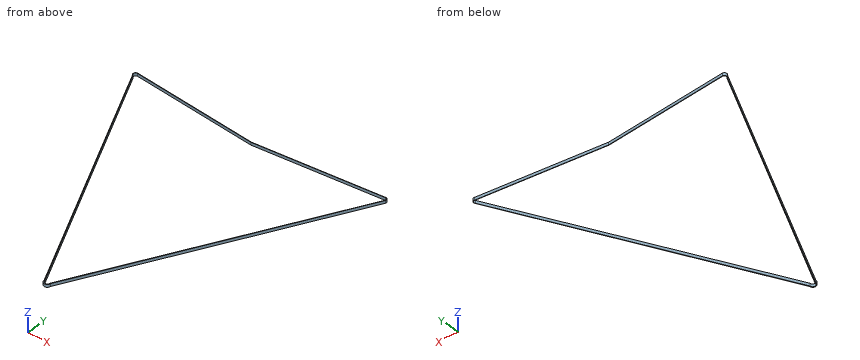
Autodesk Inventor part; units mm, degrees
ref_plane "YZ Plane" through (0, 0, 0) normal (1, 0, 0) x (0, 1, 0)
ref_plane "XZ Plane" through (0, 0, 0) normal (0, 1, 0) x (-1, 0, 0)
ref_plane "XY Plane" through (0, 0, 0) normal (0, 0, 1) x (1, 0, 0)
sketch "Sketch1" plane through (0, 0, 0) normal (0, 0, 1) x (1, 0, 0)
  arc A0 (-287.0527, -558.563) -> (-272.0536, -558.5587) centre (-279.5531, -558.6452) ccw
  line L0 (-561.7795, -4.4916) -> (-287.0527, -558.563)
  line L1 (-272.0536, -558.5587) -> (6.4474, -0.1094)
  line L2 (-0.0123, 6.4539) -> (-558.6713, 5.3904)
  arc A1 (-558.6713, 5.3904) -> (-561.7795, -4.4916) centre (-558.6609, -0.0427) ccw
  arc A2 (6.4474, -0.1094) -> (-0.0123, 6.4539) centre (1.1622, 1.1493) ccw
  point P0 (0, 0)
  dimension "d0" = 5.433
extrude "Extrusion1" add sketch "Sketch1" along normal blind 6
sketch "Sketch3" plane through (0, 0, 6) normal (0, 0, 1) x (1, 0, 0)
  line L0 (-561.7795, -4.4916) -> (-287.0527, -558.563)
  arc A0 (-287.0527, -558.563) -> (-272.0536, -558.5587) centre (-279.5531, -558.6452) ccw
  line L1 (-272.0536, -558.5587) -> (6.4474, -0.1094)
  arc A1 (6.4474, -0.1094) -> (-0.0123, 6.4539) centre (1.1622, 1.1493) ccw
  line L2 (-0.0123, 6.4539) -> (-558.6713, 5.3904)
  arc A2 (-558.6713, 5.3904) -> (-561.7795, -4.4916) centre (-558.6609, -0.0427) ccw
  line L3 (-0.0123, 6.4539) -> (-279.291, -20.76)
  line L4 (-0.0123, 6.4539) -> (-558.6713, 5.3904)
  line L5 (-279.291, -20.76) -> (-558.6713, 5.3904)
  line L6 (-558.6713, 5.3904) -> (-279.551, 142.5192)
  line L7 (-279.551, 142.5192) -> (-0.0123, 6.4539)
  point P0 (0, 0)
extrude "Extrusion2" cut sketch "Sketch3" against normal blind 6 contours L6 L7 L2 | L2 L3 L5
sketch "Sketch4" plane through (0, 0, 6) normal (0, 0, 1) x (1, 0, 0)
  point P0 (0, 0)
sketch "Sketch5" plane through (0, 0, 6) normal (0, 0, 1) x (1, 0, 0)
  line L0 (-0.0123, 6.4539) -> (-279.291, -20.76)
  line L1 (-279.291, -20.76) -> (-558.6713, 5.3904)
  arc A0 (-558.6713, 5.3904) -> (-561.7795, -4.4916) centre (-558.6609, -0.0427) ccw
  line L2 (-561.7795, -4.4916) -> (-287.0527, -558.563)
  arc A1 (-287.0527, -558.563) -> (-272.0536, -558.5587) centre (-279.5531, -558.6452) ccw
  line L3 (-272.0536, -558.5587) -> (6.4474, -0.1094)
  arc A2 (6.4474, -0.1094) -> (-0.0123, 6.4539) centre (1.1622, 1.1493) ccw
  arc A3 (-285.3025, -558.563) -> (-273.8037, -558.563) centre (-279.5531, -558.6452) ccw
  arc A4 (5.0344, -1.1313) -> (0.2947, 5.5587) centre (1.1622, 1.1493) ccw
  arc A5 (-558.1379, 4.3653) -> (-560.7286, -3.9705) centre (-558.6609, -0.0427) ccw
  line L4 (-560.7286, -3.9705) -> (-285.3025, -558.563)
  line L5 (-273.8037, -558.563) -> (5.0344, -1.1313)
  line L6 (1.1622, 5.6432) -> (-279.5531, -21.7107)
  line L7 (-279.5531, -21.7107) -> (-558.1379, 4.3653)
  point P0 (0, 0)
  dimension "d5" = 11.5
extrude "Extrusion3" cut sketch "Sketch5" against normal blind 6 contours L4 A5 L7 L6 A4 L5 A3
properties part number "z bELT"
The model under review builds one solid part; all positions refer to its coordinate system, in mm. Coordinates: 2 decimals unless noted, no trailing zeros. Order: outer loops, then holes, each group sorted by start corner. A loop starts at its lowest first (then second) coordinate and runs counter-clockwise, first axis right, second up. Notation, with made-up numbers: M 68.5,-16.5 L 78.5,-16.5 A22 ccw 78.5,-0.5 Z; hole C -31.75,-39 d7. An arc over 180 degrees is marked long. One line per question, with ' | ' between items.
(1) For probe 1 along Y at (x, z) = (-272, 2.6); probe 2 along Y at (x, z) = (-294, 1.75); probe 3 along X at (y, z) = (-82, 4.6), list the stretches that pass through material, from the lowest coordinate up. Write a range as from..to.
Geometry results:
probe 1: y = -558.45..-554.96, -20.97..-20.05 | probe 2: y = -544.55..-541.05, -20.36..-19.38 | probe 3: x = -523.35..-521.98, -35.42..-34.39
(2) Add section C-C, the plane y = -111. Write out the cut boundary in (x, z), then the cut area to 3 significant figures.
Geometry results:
outline: M -508.97,0 L -507.57,0 L -507.57,6 L -508.97,6 Z; M -49.92,0 L -48.85,0 L -48.85,6 L -49.92,6 Z | area: 14.8 mm²
(3) Add section B-B, the plane x = -71.5. Write out the cut boundary in (y, z).
Geometry results:
outline: M -156.41,0 L -154.13,0 L -154.13,6 L -156.41,6 Z; M -1.44,0 L -0.51,0 L -0.51,6 L -1.44,6 Z
(4) Add section A-A, the plane z = 2.1. Write out the cut boundary in (x, y), then the cut area to 3 significant figures.
Geometry results:
outline: M -561.78,-4.49 L -287.05,-558.56 A7.5 ccw long -272.05,-558.56 L 6.45,-0.11 A5.43 ccw -0.01,6.45 L -279.29,-20.76 L -558.67,5.39 A5.43 ccw Z; hole M -560.73,-3.97 L -285.3,-558.56 A5.75 ccw long -273.8,-558.56 L 5.03,-1.13 A4.49 ccw 1.16,5.64 L -279.55,-21.71 L -558.14,4.37 A4.44 ccw Z | area: 2,180 mm²
(5) Insertion check: pin 1 (1.5 mm diameter, centred on y = -447.5, z = 4.5, fed in from -X); pin 2 (1 mm diameter, centred on x = -200.5, z = 4.5, fed in from -Y); pin 3 (3 mm diameter, centred on y = -75.5, z = 1.5, fed in from -X). Each pin has a flat end and moves straight along its axis. Give the tip position at first contact, or say it passes through.
Geometry results:
pin 1: stops at x = -342.49 | pin 2: stops at y = -416.08 | pin 3: stops at x = -527.31
